The listing builds one solid part. Answer for the finished solid, in the listing's coordinates (mm). A direction names the side the tool comes from. Round coordinates to 2 decimals unless told otherwise and drop trailing zeros. Write each loop counter-clockwise with the first axis right and the second up, starting at its lowest first coordinate (ties: lowest second). Pieces come first, ordered by that corner, then holes.
(1) Each of these flat-tipped pins is pushed along its axis until it touches: pin 1 Ø2 at (x, z) = (-17, 26) entering from +Y; pin 2 Ø2 at (x, z) = (-7, 21.5) entering from +Y; pin 3 Ø1 at (x, z) = (-4.5, 6.5) entering from -Y. Where does it stop, or does it pass through?
(2) The mould has two halves that part along X. Classify faces 5 (the face through (9.97, 30.76, 24.75)), 6 (the face through (-3.255, 54.787, 16.224)), 7 (the face through (0, 47, 26)), 8 (the face through (-8, -20, 16)): +X half, -X half, draft (parallel to the pull), parting line (faces both ways), or undercut.
(3) A cutting plane is placed at B-B, the plane z = 29. Give the vertices of the cut face in (x, y).
(4) Find the intervals of material crossed by probe 1 along X at (y, z) = (30, 23); probe 2 along Y at (x, z) = (0, 23); probe 3 along Y at (x, z) = (0, 15), in increasing order.
(5) A cutting plane is placed at C-C, the plane y = 3. Give the vertices of the cut face in (x, z).
(6) For faces 1 (the face through (6, -20, 11)), 2 (the face through (-9.6, -1, 3)), 3 (the face through (6, 46, 29)), 4 (the face through (-12, -20, 14)), determine the directions among +Z, -Z, +X, -X, +Y, -Y from which every point of the face is accessible in a straight line to the end or side of a thin tool.
(7) A cutting plane is placed at D-D, the plane x = 2. Give the vertices of the cut face in (y, z), and give its area (3 significant figures).
(8) A cutting plane is placed at A-A, the plane y = -20.5. Give the vertices of the cut face in (x, z).
Autodesk Inventor part; units mm, degrees
ref_plane "YZ Plane" through (0, 0, 0) normal (1, 0, 0) x (0, 1, 0)
ref_plane "XZ Plane" through (0, 0, 0) normal (0, 1, 0) x (-1, 0, 0)
ref_plane "XY Plane" through (0, 0, 0) normal (0, 0, 1) x (1, 0, 0)
sketch "Sketch1" plane through (0, 0, 0) normal (0, 0, 1) x (1, 0, 0)
  line L0 (-25, 30) -> (25, 30)
  line L1 (25, 30) -> (25, -30)
  line L2 (25, -30) -> (-25, -30)
  line L3 (-25, -30) -> (-25, 30)
  line L4 (-25, 30) -> (25, -30) construction
  line L5 (25, 30) -> (-25, -30) construction
  arc A0 (-25, -30) -> (25, -30) centre (0, -30) ccw
  point P0 (0, 0)
  dimension "d0" = 50
  dimension "d1" = 60
  dimension "d2" = 25
extrude "Extrusion1" add sketch "Sketch1" along normal blind 12
sketch "Sketch2" plane through (0, 0, 12) normal (0, 0, 1) x (1, 0, 0)
  line L0 (25, 30) -> (-25, 30)
  circle A0 centre (0, 30) radius 25
  point P0 (0, 0)
  dimension "d5" = 50
extrude "Extrusion2" add sketch "Sketch2" along normal blind 20 and the other way blind 12
sketch "Sketch3" plane through (0, 30, 32) normal (0, 0, 1) x (1, 0, 0)
  line L0 (-6, -25) -> (6, -25)
  line L1 (6, 25) -> (-6, 25)
  line L2 (-6, -25) -> (6, 25) construction
  line L3 (6, -25) -> (-6, 25) construction
  line L4 (-6, 25) -> (-6, 8)
  line L5 (-6, -8) -> (-6, -25)
  line L6 (6, -25) -> (6, -8)
  line L7 (6, 8) -> (6, 25)
  arc A0 (-6, 8) -> (-6, -8) centre (0, 0) ccw
  arc A1 (6, -8) -> (6, 8) centre (0, 0) ccw
  point P0 (0, -30)
  dimension "d11" = 12
  dimension "d12" = 50
extrude "Extrusion3" cut sketch "Sketch3" against normal blind 6
sketch "Sketch4" plane through (0, 30, 26) normal (0, 0, 1) x (1, 0, 0)
  arc A0 (6, -8) -> (6, 8) centre (0, 0) ccw
  circle A1 centre (0, 0) radius 10
  point P0 (0, -30)
  point P1 (6, 8)
  point P2 (6, -8)
  dimension "d15" = 20
extrude "Extrusion4" cut sketch "Sketch4" against normal blind 6
sketch "Sketch5" plane through (0, 0, 12) normal (0, 0, 1) x (1, 0, 0)
  arc A0 (-25, -30) -> (25, -30) centre (0, -30) ccw
  line L0 (0, -30) -> (0, -10) construction
  line L1 (12, -30) -> (12, -10)
  line L2 (-12, -10) -> (-12, -30)
  arc A1 (-12, -30) -> (12, -30) centre (0, -30) ccw
  arc A2 (12, -10) -> (-12, -10) centre (0, -10) ccw
  line L3 (-6, -10) -> (-6, -30)
  arc A3 (-6, -30) -> (6, -30) centre (0, -30) ccw
  line L4 (6, -30) -> (6, -10)
  arc A4 (6, -10) -> (-6, -10) centre (0, -10) ccw
  point P0 (0, 0)
  point P1 (0, -20)
  dimension "d21" = 12
  dimension "d22" = 6
extrude "Extrusion5" add sketch "Sketch5" along normal blind 4
sketch "Sketch6" plane through (0, 0, 0) normal (0, 1, 0) x (-1, 0, 0)
  line L0 (-25, 0) -> (25, 0)
  line L1 (-10.3999, 0) -> (9.6001, 0)
  line L2 (9.6001, 0) -> (9.6001, 6)
  line L3 (9.6001, 6) -> (-10.3999, 6)
  line L4 (-10.3999, 6) -> (-10.3999, 0)
  point P0 (0, 0)
  point P1 (9.6001, 0)
  dimension "d25" = 20
  dimension "d26" = 6
extrude "Extrusion6" cut sketch "Sketch6" along normal blind 60 and the other way blind 60
sketch "Sketch7" plane through (0, 0, 12) normal (0, 0, 1) x (1, 0, 0)
  arc A0 (6, -10) -> (-6, -10) centre (0, -10) ccw
  line L0 (0, -4) -> (0, -36) construction
  arc A1 (-6, -30) -> (6, -30) centre (0, -30) ccw
  line L1 (6, -10) -> (6, -30)
  line L2 (-6, -30) -> (-6, -10)
  arc A2 (6, -10) -> (-6, -10) centre (0, -10) ccw
  arc A3 (-6, -30) -> (6, -30) centre (0, -30) ccw
  point P0 (0, 0)
  point P1 (0, -20)
extrude "Extrusion7" cut sketch "Sketch7" against normal through all
properties part number "cad@67"
Solutions:
1. pin 1: stops at y = 49.21
1. pin 2: stops at y = 54.27
1. pin 3: stops at y = -54.68
2. face 5: undercut
2. face 6: parting line
2. face 7: undercut
2. face 8: draft
3. outline: (-6, 5.73) - (-6, 22) arc R10 cw to (-6, 38) - (-6, 54.27) arc R25 ccw to start; (6, 5.73) arc R25 ccw to (6, 54.27) - (6, 38) arc R10 cw to (6, 22) - close
4. probe 1: x = -25 to -10, 10 to 25
4. probe 2: y = 5 to 20, 40 to 55
4. probe 3: y = -42 to -36, -4 to 2, 5 to 55
5. outline: (-25, 0) - (-9.6, 0) - (-9.6, 6) - (10.4, 6) - (10.4, 0) - (25, 0) - (25, 12) - (-25, 12) - close
6. face 1: +Z, -Z
6. face 2: -Z, +Y, -Y
6. face 3: +Z, +Y, -Y
6. face 4: +Z, -X, -Y
7. outline: (-54.92, 6) - (-35.66, 6) - (-35.66, 16) - (-41.83, 16) - (-41.83, 12) - (-54.92, 12) - close; (-4.34, 6) - (54.92, 6) - (54.92, 26) - (39.8, 26) - (39.8, 20) - (20.2, 20) - (20.2, 26) - (5.08, 26) - (5.08, 12) - (1.83, 12) - (1.83, 16) - (-4.34, 16) - close
7. area: 1,100 mm2
8. outline: (-25, 0) - (-9.6, 0) - (-9.6, 6) - (-6, 6) - (-6, 16) - (-12, 16) - (-12, 12) - (-25, 12) - close; (6, 6) - (10.4, 6) - (10.4, 0) - (25, 0) - (25, 12) - (12, 12) - (12, 16) - (6, 16) - close
